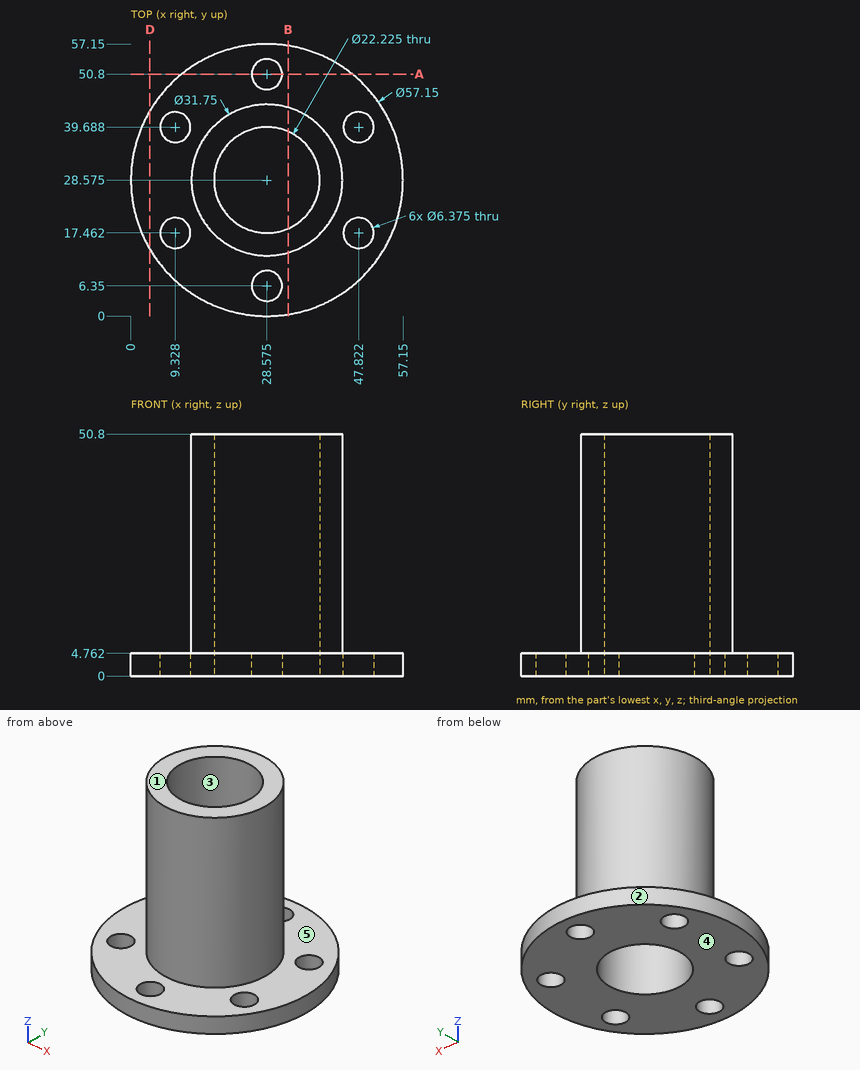
Here's the drawing with two shaded views (mm, measured from the low corner). I have some questions. A direction names the side the tool comes from. Give positions to 0.01 mm unless a question says otherwise; leave off trailing zeros. Order: outer loops, then holes, each group sorted by start corner. A loop starts at its lowest first (then second) coordinate and runs counter-clockwise, first axis right, second up. Notation, with made-up numbers: M 45.5,29 L 74.5,29 A13 ccw 74.5,35 Z; hole C 77,-39 d9. An arc over 180 degrees is marked long. Answer as a JSON object with one key per item and string values. Group by question number.
1) We'd pull the mould along Y, two halves only. Please class the marked faces 1, 2 and 3: pulls with the +Y half, pulls with the -Y half, needs draft (parallel to the pull), parting line crosses it, or undercut.
2) On a 3-axis mill with a long thin cutter (end or side, diameter ignored), from which of +Z, -Z, +X, -X, +Y, -Y can I reach the whole of each face in a straight line? I mean the marked faces 4 and 5. Say none if no direction works.
3) Suppose I cut it at B-B, the plane x = 33. Write out the boundary of the cut face in (y, z) (1 decimal), plus the area to 3 significant figures.
4) Please list where these lines run through material, in increasing order: L1, parallel to Y at x = 28.5, z = 3.5; L2, parallel to Z at x = 14, y = 38.5; L3, parallel to X at y = 29, z = 3. Write a range as [from, to].
5) Suppose I cut it at D-D, the plane x = 4. Write out the boundary of the cut face in (y, z) (1 decimal).
6) I'm going to push flat-ended pins straight in: pin 1 Ø5 at (y, z) = (28.5, 16) entering from -X; pin 2 Ø4 at (x, y) = (9.33, 17.46) entering from +Z; pin 3 Ø12 at (y, z) = (14, 30.5) entering from +X (1 decimal); pin 4 Ø2 at (x, z) = (29.5, 26.5) entering from +Y. Where does each tip first touch, or does it pass through?
7) Suppose I cut it at A-A, the plane y = 50.8. Write out the boundary of the cut face in (x, z) (1 decimal).
Results found:
{
 "1": {"face 1": "needs draft", "face 2": "parting line crosses it", "face 3": "undercut"},
 "2": {"face 4": "-Z, +X, -X, +Y, -Y", "face 5": "+Z"},
 "3": {"outline": "M 0.3,0 L 18.4,0 L 18.4,50.8 L 13.3,50.8 L 13.3,4.8 L 0.3,4.8 Z; M 38.8,0 L 56.8,0 L 56.8,4.8 L 43.8,4.8 L 43.8,50.8 L 38.8,50.8 Z", "area": "637 mm²"},
 "4": {"L1": "[0, 3.16], [9.54, 17.46], [39.69, 47.61], [53.99, 57.15]", "L2": "[0, 4.76]", "L3": "[0, 17.47], [39.68, 57.15]"},
 "5": {"outline": "M 14,0 L 43.2,0 L 43.2,4.8 L 14,4.8 Z"},
 "6": {"pin 1": "x = 12.7", "pin 2": "through", "pin 3": "x = 41.9", "pin 4": "y = 44.45"},
 "7": {"outline": "M 10.6,0 L 25.4,0 L 25.4,4.8 L 10.6,4.8 Z; M 31.8,0 L 46.5,0 L 46.5,4.8 L 31.8,4.8 Z"}
}
